The model under review builds one solid part; all positions refer to its coordinate system, in mm. A direction names the side the tool comes from. Coordinates: 2 decimals unless noted, no trailing zeros. Write each loop counter-clockwise with the first axis right and the second up, starting at its lowest first coordinate (ties: lowest second). Pieces come first, ordered by that corner, then holes. Notation, with made-up numbers: M -10.5,-40 L 2.5,-40 A17 ccw 2.5,-34 Z; hole C 66,27 d4. An arc over 180 degrees is marked long. Answer as a JSON object with one key per item and string values.
```python
from build123d import *

# Parameters (mm, degrees)
F0_R      = 65
F1_DEPTH  = 15
F2_W      = 3
F2_H      = 70
F3_DEPTH  = 25
F5_DEPTH  = 3
F7_D      = 5
F8_R      = 3
F8_R_2    = 2.5
F9_DEPTH  = 10
F10_R     = 3
F11_DEPTH = 10
F12_R     = 3
F13_DEPTH = 10.1
F14_R     = 3
F15_DEPTH = 10


with BuildPart() as f1:
    # F0 (on Top) → F1 (new body)
    with BuildSketch(Plane.XY):
        Circle(F0_R)
    extrude(amount=F1_DEPTH)

    # F2 (on face) → F3 (join)
    with BuildSketch(Plane.XY.offset(15)):
        with Locations((-6.5, 0)):
            Rectangle(F2_W, F2_H)
    extrude(amount=F3_DEPTH)

    # F4 (on face) → F5 (join)
    with BuildSketch(Plane(origin=(-8, 0, 0), x_dir=(0, -1, 0), z_dir=(-1, 0, 0))):
        Polygon((-35, 40), (35, 40), (-10.6395371258, 61.74890697), align=None)
    extrude(amount=-F5_DEPTH)

    # F7 (through all)
    with Locations(Plane(origin=(-8, 0, 0), x_dir=(0, -1, 0), z_dir=(-1, 0, 0))):
        with Locations((-2.5252789198, 46.2088645364), (24.5568976072, 33.3032179211)):
            Hole(F7_D / 2)

    # F8 (on face) → F9 (join)
    with BuildSketch(Plane.YZ.offset(-5)):
        Polygon((-32.0568976072, 295.8032179211), (-32.0568976072, 41.4024958221), (-17.0568976072, 48.5505438764), (-17.0568976072, 295.8032179211), align=None)
        with Locations((-24.5568976072, 288.3032179211)):
            Circle(F8_R, mode=Mode.SUBTRACT)
        Polygon((-4.9747210802, 308.7088645364), (-4.9747210802, 54.3081424374), (10.0252789198, 61.4561904917), (10.0252789198, 308.7088645364), (2.5252789198, 308.7088645364), align=None)
        with BuildLine():
            ThreePointArc((5.5252789198, 301.2088645364), (0.4039585762, 299.0875441928), (2.5252789198, 304.2088645364))
            ThreePointArc((2.5252789198, 304.2088645364), (4.6465992633, 303.3301848799), (5.5252789198, 301.2088645364))
        make_face(mode=Mode.SUBTRACT)
        Polygon((10.0252789198, 61.4561904917), (-4.9747210802, 54.3081424374), (-4.9747210802, 38.7088645364), (10.0252789198, 38.7088645364), align=None)
        with Locations((2.5252789198, 46.2088645364)):
            Circle(F8_R_2, mode=Mode.SUBTRACT)
        Polygon((-32.0568976072, 41.4024958221), (-32.0568976072, 25.8032179211), (-17.0568976072, 25.8032179211), (-17.0568976072, 48.5505438764), align=None)
        with Locations((-24.5568976072, 33.3032179211)):
            Circle(F8_R_2, mode=Mode.SUBTRACT)
    extrude(amount=F9_DEPTH)

    # F10 (on face) → F11 (join)
    with BuildSketch(Plane(origin=(-5, 0, 0), x_dir=(0, -1, 0), z_dir=(-1, 0, 0))):
        with BuildLine():
            Line((36.9886778951, 289.224208002), (34.7282933681, 317.885416384))
            ThreePointArc((34.7282933681, 317.885416384), (28.1753092515, 329.1496679175), (15.161757221, 328.4623346707))
            Line((15.161757221, 328.4623346707), (-8.9063381185, 311.9574497225))
            Line((-8.9063381185, 311.9574497225), (-10.2528547102, 311.03406542))
            ThreePointArc((-10.2528547102, 311.03406542), (-14.9500569426, 299.8395979138), (-7.9278259355, 289.9366648512))
            Line((-7.9278259355, 289.9366648512), (18.9534333664, 277.0529978406))
            Line((18.9534333664, 277.0529978406), (19.2974731878, 276.8881062168))
            ThreePointArc((19.2974731878, 276.8881062168), (31.6770683616, 277.9880576803), (36.9886778951, 289.224208002))
        make_face()
        with Locations((-2.5252789198, 301.2088645364)):
            Circle(F10_R, mode=Mode.SUBTRACT)
        with Locations((24.5273711722, 288.2414390787)):
            Circle(F10_R, mode=Mode.SUBTRACT)
        with Locations((22.2311670236, 318.1534334177)):
            Circle(F10_R, mode=Mode.SUBTRACT)
    extrude(amount=F11_DEPTH)

    # F12 (on face) → F13 (join)
    with BuildSketch(Plane.YZ.offset(-5)):
        with BuildLine():
            Line((-287.0568976072, 280.7414390787), (-34.5273711722, 280.7414390787))
            ThreePointArc((-34.5273711722, 280.7414390787), (-36.5322417286, 284.7581815627), (-36.9886778951, 289.224208002))
            Line((-36.9886778951, 289.224208002), (-36.4698200708, 295.8032179211))
            Line((-36.4698200708, 295.8032179211), (-287.0568976072, 295.8032179211))
            Line((-287.0568976072, 295.8032179211), (-287.0568976072, 280.7414390787))
        make_face()
        with Locations((-279.5568976072, 288.2723284999)):
            Circle(F12_R, mode=Mode.SUBTRACT)
        with BuildLine():
            Line((-284.6566983312, 310.7544099386), (-35.2906847515, 310.7544099386))
            Line((-35.2906847515, 310.7544099386), (-34.7282933681, 317.885416384))
            ThreePointArc((-34.7282933681, 317.885416384), (-34.09968308, 322.0762291833), (-32.1070052282, 325.816188781))
            Line((-32.1070052282, 325.816188781), (-284.6566983312, 325.816188781))
            Line((-284.6566983312, 325.816188781), (-284.6566983312, 310.7544099386))
        make_face()
        with Locations((-277.1566983312, 318.2852993598)):
            Circle(F12_R, mode=Mode.SUBTRACT)
        with BuildLine():
            Line((-34.5273711722, 280.7414390787), (-32.0568976072, 280.7414390787))
            Line((-32.0568976072, 280.7414390787), (-32.0568976072, 295.8032179211))
            Line((-32.0568976072, 295.8032179211), (-36.4698200708, 295.8032179211))
            Line((-36.4698200708, 295.8032179211), (-36.9886778951, 289.224208002))
            ThreePointArc((-36.9886778951, 289.224208002), (-36.5322417286, 284.7581815627), (-34.5273711722, 280.7414390787))
        make_face()
        with BuildLine():
            Line((-34.7282933681, 317.885416384), (-35.2906847515, 310.7544099386))
            Line((-35.2906847515, 310.7544099386), (-14.6566983312, 310.7544099386))
            Line((-14.6566983312, 310.7544099386), (-14.6566983312, 325.816188781))
            Line((-14.6566983312, 325.816188781), (-32.1070052282, 325.816188781))
            ThreePointArc((-32.1070052282, 325.816188781), (-34.09968308, 322.0762291833), (-34.7282933681, 317.885416384))
        make_face()
        with Locations((-22.2311670236, 318.1534334177)):
            Circle(F12_R, mode=Mode.SUBTRACT)
    extrude(amount=F13_DEPTH)

    # F14 (on face) → F15 (join)
    with BuildSketch(Plane(origin=(-5, 0, 0), x_dir=(0, -1, 0), z_dir=(-1, 0, 0))):
        with BuildLine():
            ThreePointArc((267.0595581049, 287.1736825743), (267.8604330049, 283.7810187252), (269.5670449033, 280.7414390787))
            Line((269.5670449033, 280.7414390787), (287.0568976072, 280.7414390787))
            Line((287.0568976072, 280.7414390787), (287.0568976072, 295.8032179211))
            Line((287.0568976072, 295.8032179211), (266.3966875062, 295.8032179211))
            Line((266.3966875062, 295.8032179211), (267.0303385293, 287.5540756116))
            Line((267.0303385293, 287.5540756116), (267.0595581049, 287.1736825743))
        make_face()
        with BuildLine():
            ThreePointArc((277.43915398, 286.1474374605), (277.3573466714, 290.4139524214), (281.6245254003, 290.446015531))
            ThreePointArc((281.6245254003, 290.446015531), (282.3139688231, 289.4549350745), (282.5568976072, 288.2723284999))
            ThreePointArc((282.5568976072, 288.2723284999), (280.7072821339, 285.5016579239), (277.43915398, 286.1474374605))
        make_face(mode=Mode.SUBTRACT)
        with BuildLine():
            Line((286.5885379882, 278.0207007669), (310.2796802866, 294.3088553806))
            ThreePointArc((310.2796802866, 294.3088553806), (316.758316211, 305.6160318629), (309.6562921431, 316.5424318913))
            Line((309.6562921431, 316.5424318913), (283.3285948217, 329.133571402))
            Line((283.3285948217, 329.133571402), (281.8556622624, 329.8379968258))
            ThreePointArc((281.8556622624, 329.8379968258), (269.812367904, 328.3086595327), (264.7472918034, 317.275762558))
            Line((264.7472918034, 317.275762558), (266.3966875062, 295.8032179211))
            Line((266.3966875062, 295.8032179211), (287.0568976072, 295.8032179211))
            Line((287.0568976072, 295.8032179211), (287.0568976072, 280.7414390787))
            Line((287.0568976072, 280.7414390787), (269.5670449033, 280.7414390787))
            ThreePointArc((269.5670449033, 280.7414390787), (277.5338100054, 275.9778112248), (286.5885379882, 278.0207007669))
        make_face()
        with Locations((304.2632266742, 305.2656927861)):
            Circle(F14_R, mode=Mode.SUBTRACT)
        with Locations((277.2105765951, 318.2331194398)):
            Circle(F14_R, mode=Mode.SUBTRACT)
    extrude(amount=F15_DEPTH)


solid = f1.part
```
(1) Add section D-D on x = 48.5. Give the boundary of the cut face in (y, z).
Results list:
{"outline": "M -43.28,0 L 43.28,0 L 43.28,15 L -43.28,15 Z"}
(2) Add section A-A on z = 223. Give the boundary of the cut face in (x, y), and give its area (3 significant figures).
Results list:
{"outline": "M -5,-32.06 L 5,-32.06 L 5,-17.06 L -5,-17.06 Z; M -5,-4.97 L 5,-4.97 L 5,10.03 L -5,10.03 Z", "area": "300 mm²"}
(3) For faces 1 (the face through (-9.93, -316.762, 305.424)), 2 (the face through (-9.93, -35.874, 303.354)), 3 (the face through (0, -148, 325.816)), 4 (the face through (0, -287.057, 288)), 5 (the face through (-9.93, -31.527, 277.885)), list the 3-axis set-ups (+Z, -Z, +X, -X, +Y, -Y) from which the entire face can be reached by the end or side of a thin tool; tool diameter is ignored.
Results list:
{"face 1": "+X, -X, -Y", "face 2": "+Z, -X", "face 3": "+Z, +X, +Y, -Y", "face 4": "+Z, -Z, +X, -Y", "face 5": "-X"}
(4) Draft analysis for pull direction Y (two halves, no side actions). For faces 6 (the face through (-6.521, 22.649, 51.027)), 7 (the face through (0, -17.057, 159)), 8 (the face through (-15, -16, 304)), 9 (the face through (-6.52, -12.5, 50.72)), state which applies: released by +Y, released by -Y, zero draft, split by the parting line, or undercut.
Results list:
{"face 6": "released by +Y", "face 7": "undercut", "face 8": "zero draft", "face 9": "released by -Y"}
(5) Add section B-B on y = -253.5. Give the boundary of the cut face in (x, z), and give its area (3 significant figures).
Results list:
{"outline": "M -5,280.74 L 5.1,280.74 L 5.1,295.8 L -5,295.8 Z; M -5,310.75 L 5.1,310.75 L 5.1,325.82 L -5,325.82 Z", "area": "304 mm²"}
(6) For pin 1 Ø6.5 at (y, z) = (2.53, 46.21) entering from +X; pin 2 Ø10 at (x, z) = (4, 229) entering from -Y; pin 3 Ø8 at (x, z) = (2, 97.5) entering from +Y, all flat-tipped, find the tip position at first contact; note any pin that passes through.
Results list:
{"pin 1": "x = 5", "pin 2": "y = -32.06", "pin 3": "y = 10.03"}
(7) Add section C-C on x = 0. Count the separate pieces of the cut face and the enclosed holes in it, and give its area (3 significant figures).
Results list:
{"separate pieces": "4", "enclosed holes": "7", "area": "17,800 mm²"}
(8) Wall thickness on line 1 along Z through (x, y) = (18.5, 4.5); line 2 along Y through (x, z) = (1, 90); line 3 along Z through (x, y) = (1, -274): over which ranges is each line inside the solid? List them lowest first. Write a range as from..to.
Results list:
{"line 1": "0..15", "line 2": "-32.06..-17.06, -4.97..10.03", "line 3": "280.74..295.8, 310.75..325.82"}
